from build123d import *

# Parameters (mm, degrees)
PAD_DEPTH    = 3.775
SKETCH001_W  = 6.69
SKETCH001_H  = 0.7
POCKET_DEPTH = 5
FILLET_R     = 0.3
FILLET001_R  = 0.3


with BuildPart() as part:
    # Sketch → Pad (new body, symmetric)
    with BuildSketch(Plane.XZ):
        with BuildLine():
            Line((-3.17, 3.26), (3.17, 3.26))
            ThreePointArc((4.47, 1.96), (4.089239, 2.879239), (3.17, 3.26))
            Line((4.47, 1.96), (4.47, 1.3))
            ThreePointArc((3.17, 0), (4.089239, 0.380761), (4.47, 1.3))
            Line((3.17, 0), (-3.17, 0))
            ThreePointArc((-4.47, 1.3), (-4.089239, 0.380761), (-3.17, 0))
            Line((-4.47, 1.3), (-4.47, 1.96))
            ThreePointArc((-3.17, 3.26), (-4.089239, 2.879239), (-4.47, 1.96))
        make_face()
    extrude(amount=PAD_DEPTH, both=True)

    # Sketch001 (on Face10 of Pad) → Pocket (cut)
    with BuildSketch(Plane.XZ.offset(3.775)):
        with BuildLine():
            Line((-3.17, 2.96), (3.17, 2.96))
            ThreePointArc((4.17, 1.96), (3.877107, 2.667107), (3.17, 2.96))
            Line((4.17, 1.96), (4.17, 1.3))
            ThreePointArc((3.17, 0.3), (3.877107, 0.592893), (4.17, 1.3))
            Line((3.17, 0.3), (-3.17, 0.3))
            ThreePointArc((-4.17, 1.3), (-3.877107, 0.592893), (-3.17, 0.3))
            Line((-4.17, 1.3), (-4.17, 1.96))
            ThreePointArc((-3.17, 2.96), (-3.877107, 2.667107), (-4.17, 1.96))
        make_face()
        with Locations((0.107557, 1.579315)):
            Rectangle(SKETCH001_W, SKETCH001_H, mode=Mode.SUBTRACT)
    extrude(amount=-POCKET_DEPTH, mode=Mode.SUBTRACT)

    # Fillet
    fillet_edges = [part.edges().sort_by_distance(p)[0] for p in [
        (3.452557, -1.275, 1.229315),
        (3.452557, -1.275, 1.929315),
        (-3.237443, -1.275, 1.929315),
        (-3.237443, -1.275, 1.229315),
    ]]
    fillet(fillet_edges, radius=FILLET_R)

    # Fillet001
    fillet001_edges = [part.edges().sort_by_distance(p)[0] for p in [
        (0.107557, -3.775, 1.229315),
        (3.364689, -3.775, 1.317183),
        (-3.149575, -3.775, 1.317183),
        (3.452557, -3.775, 1.579315),
        (-3.237443, -3.775, 1.579315),
        (3.364689, -3.775, 1.841447),
        (-3.149575, -3.775, 1.841447),
        (0.107557, -3.775, 1.929315),
    ]]
    fillet(fillet001_edges, radius=FILLET001_R)


solid = part.part
Build history of the part. All positions in model axes, mm. A direction names the side the tool comes from. Round coordinates to 2 decimals unless told otherwise and drop trailing zeros. Loops run counter-clockwise (first coordinate to the right, second up) from the corner with the lowest first, then second, coordinate; pieces in that order, holes last. Notation, with made-up numbers: (30.25, -20) -> (59.25, -20) arc R22 ccw to (59.25, 2) -> close; hole circle Ø3 at (33, 87). An arc over 180 degrees is marked (long way). One line per item, written item: value. Start each with the question number.
Q1. Cut at C-C on y = 2. List the corners of the cut face in (x, z), plus the area to 3 significant figures.
Q2. Cut at A-A on y = -2.25. List the corners of the cut face in (x, z), plus the area to 3 significant figures.
Q3. Probe line 1 along Z through (x, y) = (-2, 0.5); line 2 along X through (y, z) = (0.25, 1.45); line 3 along X through (y, z) = (-3, 0.55). List the from-to ranges inside material, lowest first.
Q4. Cut at D-D on z = 2.7. List the corners of the cut face in (x, y) (3 decimals), plus the area to 3 significant figures.
Q5. Two-plate mould, pull along X, no slides. Class faces 1 (the face through (-4.1, -0.05, 0.39)), 2 (the face through (0.1, 1.225, 2.2)), 3 (the face through (0, 3.775, 2)), 4 (the face through (-3.869, -1.31, 2.675)): released by +X, released by -X, zero draft, split by the parting line, or undercut.
Q6. 3-axis set-ups, long thin cutter, end or side, ignore diameter. For faces 5 (the face through (-4.08, -0.05, 2.89)), 6 (the face through (3.869, -1.31, 0.585)): which of +Z, -Z, +X, -X, +Y, -Y reach the whole face in a straight line?
Q7. Cut at B-B on x = -2.5. List the corners of the cut face in (y, z) (3 decimals), plus the area to 3 significant figures.
Computed:
1. outline: (-4.47, 1.3) arc R1.3 ccw to (-3.17, 0) -> (3.17, 0) arc R1.3 ccw to (4.47, 1.3) -> (4.47, 1.96) arc R1.3 ccw to (3.17, 3.26) -> (-3.17, 3.26) arc R1.3 ccw to (-4.47, 1.96) -> close
1. area: 27.7 mm²
2. outline: (-4.47, 1.3) arc R1.3 ccw to (-3.17, 0) -> (3.17, 0) arc R1.3 ccw to (4.47, 1.3) -> (4.47, 1.96) arc R1.3 ccw to (3.17, 3.26) -> (-3.17, 3.26) arc R1.3 ccw to (-4.47, 1.96) -> close; (-3.24, 1.53) arc R0.3 ccw to (-2.94, 1.23) -> (3.15, 1.23) arc R0.3 ccw to (3.45, 1.53) -> (3.45, 1.63) arc R0.3 ccw to (3.15, 1.93) -> (-2.94, 1.93) arc R0.3 ccw to (-3.24, 1.63) -> close; hole (-4.17, 1.3) arc R1 ccw to (-3.17, 0.3) -> (3.17, 0.3) arc R1 ccw to (4.17, 1.3) -> (4.17, 1.96) arc R1 ccw to (3.17, 2.96) -> (-3.17, 2.96) arc R1 ccw to (-4.17, 1.96) -> close
2. area: 11.0 mm²
3. line 1: 0 to 0.3, 1.23 to 1.93, 2.96 to 3.26
3. line 2: -4.47 to -4.17, -3.23 to 3.44, 4.17 to 4.47
3. line 3: -4.23 to -3.83, 3.83 to 4.23
4. outline: (-4.239, -3.775) -> (-3.843, -3.775) -> (-3.843, 1.225) -> (3.843, 1.225) -> (3.843, -3.775) -> (4.239, -3.775) -> (4.239, 3.775) -> (-4.239, 3.775) -> close
4. area: 25.6 mm²
5. face 1: released by -X
5. face 2: undercut
5. face 3: zero draft
5. face 4: undercut
6. face 5: +Z, -X, +Y, -Y
6. face 6: -Y
7. outline: (-3.775, 0) -> (3.775, 0) -> (3.775, 3.26) -> (-3.775, 3.26) -> (-3.775, 2.96) -> (1.225, 2.96) -> (1.225, 1.929) -> (-3.475, 1.929) arc R0.3 ccw to (-3.775, 1.629) -> (-3.775, 1.529) arc R0.3 ccw to (-3.475, 1.229) -> (1.225, 1.229) -> (1.225, 0.3) -> (-3.775, 0.3) -> close
7. area: 14.8 mm²
